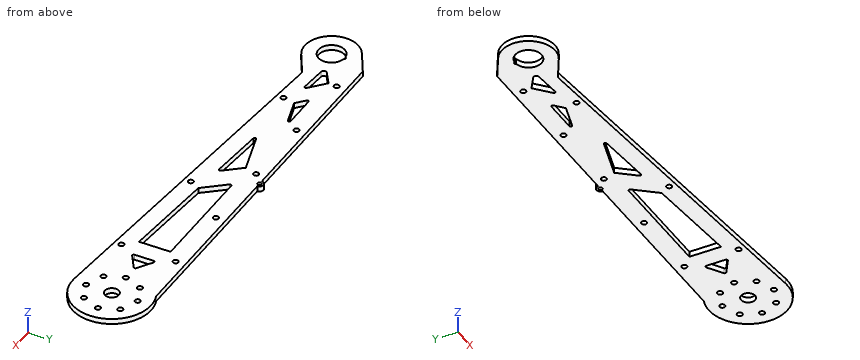
```python
from build123d import *

# Parameters (mm, degrees)
SKETCH_1_R          = 9.7
SKETCH_1_R_2        = 5.2
SKETCH_1_R_3        = 2
EXTRUDE_1_DEPTH     = 4
CUT_EXTRUDE_1_DEPTH = 10
SKETCH_3_R          = 3
EXTRUDE_2_DEPTH     = 4
SKETCH_4_R          = 1.5
CUT_EXTRUDE_2_DEPTH = 4
SKETCH_5_R          = 1
CUT_EXTRUDE_3_DEPTH = 10


with BuildPart() as part:
    # 草图1 → 凸台-拉伸1 (new body)
    with BuildSketch(Plane.XY):
        with BuildLine():
            Line((-9.85, 17.060700455), (7.470508076, 27.060700455))
            Line((7.470508076, 27.060700455), (289.624667154, 27.060700455))
            ThreePointArc((289.624667154, 27.060700455), (328.694852344, 4.11311011), (297.66555963, -28.905888469))
            Line((297.66555963, -28.905888469), (27.170508076, -7.060700455))
            Line((27.170508076, -7.060700455), (9.85, -17.060700455))
            ThreePointArc((9.85, -17.060700455), (-17.060700455, -9.85), (-9.85, 17.060700455))
        make_face()
        Circle(SKETCH_1_R, mode=Mode.SUBTRACT)
        with Locations((300, 0)):
            Circle(SKETCH_1_R_2, mode=Mode.SUBTRACT)
        with Locations((319, 0)):
            Circle(SKETCH_1_R_3, mode=Mode.SUBTRACT)
        with Locations((313.435028843, -13.435028843)):
            Circle(SKETCH_1_R_3, mode=Mode.SUBTRACT)
        with Locations((300, -19)):
            Circle(SKETCH_1_R_3, mode=Mode.SUBTRACT)
        with Locations((286.564971157, -13.435028843)):
            Circle(SKETCH_1_R_3, mode=Mode.SUBTRACT)
        with Locations((281, 0)):
            Circle(SKETCH_1_R_3, mode=Mode.SUBTRACT)
        with Locations((286.564971157, 13.435028843)):
            Circle(SKETCH_1_R_3, mode=Mode.SUBTRACT)
        with Locations((300, 19)):
            Circle(SKETCH_1_R_3, mode=Mode.SUBTRACT)
        with Locations((313.435028843, 13.435028843)):
            Circle(SKETCH_1_R_3, mode=Mode.SUBTRACT)
        with Locations((250, 20)):
            Circle(SKETCH_1_R_3, mode=Mode.SUBTRACT)
        with Locations((195, 20)):
            Circle(SKETCH_1_R_3, mode=Mode.SUBTRACT)
        with Locations((140, 20)):
            Circle(SKETCH_1_R_3, mode=Mode.SUBTRACT)
        with Locations((85, 20)):
            Circle(SKETCH_1_R_3, mode=Mode.SUBTRACT)
        with Locations((30, 20)):
            Circle(SKETCH_1_R_3, mode=Mode.SUBTRACT)
        with Locations(Location((250, -20, 0), (0, 0, 180))):
            Circle(SKETCH_1_R_3, mode=Mode.SUBTRACT)
        with Locations((167.5, -13.337297667)):
            Circle(SKETCH_1_R_3, mode=Mode.SUBTRACT)
        with Locations((57.5, -4.453694555)):
            Circle(SKETCH_1_R_3, mode=Mode.SUBTRACT)
    extrude(amount=EXTRUDE_1_DEPTH)

    # 草图2 → 切除-拉伸1 (cut)
    with BuildSketch(Plane(origin=(0, 0, 0), x_dir=(-1, 0, 0), z_dir=(0, 0, -1))):
        with BuildLine():
            Line((-137.197603441, 10.82531174), (-106.043706264, 1.591034337))
            ThreePointArc((-106.043706264, 1.591034337), (-105.333274422, 0.528665045), (-106.247395472, -0.364489265))
            Line((-106.247395472, -0.364489265), (-146.939942745, -3.650820533))
            ThreePointArc((-146.939942745, -3.650820533), (-147.907056702, -3.116572023), (-147.791851116, -2.017727835))
            Line((-147.791851116, -2.017727835), (-137.197603441, 10.82531174))
        make_face()
        with BuildLine():
            Line((-242, 12), (-159.091058121, 12))
            ThreePointArc((-159.091058121, 12), (-158.186531194, 11.426416508), (-158.319647694, 10.363662077))
            Line((-158.319647694, 10.363662077), (-171.517559676, -5.635709572))
            Line((-171.517559676, -5.635709572), (-242, -11.327873446))
            Line((-242, -11.327873446), (-242, 12))
        make_face()
        with BuildLine():
            Line((-77.967218715, 12), (-53.665101582, 12))
            ThreePointArc((-53.665101582, 12), (-52.730413268, 11.355468359), (-53.000597339, 10.252715509))
            Line((-53.000597339, 10.252715509), (-59.49167188, 4.480688084))
            Line((-59.49167188, 4.480688084), (-78.251405867, 10.041231173))
            ThreePointArc((-78.251405867, 10.041231173), (-78.956857242, 11.14358129), (-77.967218715, 12))
        make_face()
        with BuildLine():
            Line((-268.630020148, 0.840296648), (-257.54212687, 7.993776182))
            ThreePointArc((-257.54212687, 7.993776182), (-256.52152684, 8.031581712), (-256, 7.153479534))
            Line((-256, 7.153479534), (-256, -7.153479534))
            ThreePointArc((-256, -7.153479534), (-256.52152684, -8.031581712), (-257.54212687, -7.993776182))
            Line((-257.54212687, -7.993776182), (-268.630020148, -0.840296648))
            ThreePointArc((-268.630020148, -0.840296648), (-269.087893278, 0), (-268.630020148, 0.840296648))
        make_face()
        with BuildLine():
            Line((-19.631707517, 7.078552885), (-29.56189752, 13.698679554))
            Line((-29.56189752, 13.698679554), (-40.860283753, 3.651869157))
            ThreePointArc((-40.860283753, 3.651869157), (-41.116034111, 2.513264507), (-40.118555254, 1.907570918))
            Line((-40.118555254, 1.907570918), (-20.586659398, 3.4204248))
            ThreePointArc((-20.586659398, 3.4204248), (-18.805958358, 4.909282805), (-19.631707517, 7.078552885))
        make_face()
    extrude(amount=-CUT_EXTRUDE_1_DEPTH, mode=Mode.SUBTRACT)

    # 草图3 → 凸台-拉伸2 (add)
    with BuildSketch(Plane(origin=(0, 0, 0), x_dir=(-1, 0, 0), z_dir=(0, 0, -1))):
        with Locations((-148.547587615, 27.060700455)):
            Circle(SKETCH_3_R)
    extrude(amount=-EXTRUDE_2_DEPTH)

    # 草图4 → 切除-拉伸2 (cut)
    with BuildSketch(Plane(origin=(0, 0, 0), x_dir=(-1, 0, 0), z_dir=(0, 0, -1))):
        with Locations((-148.547587615, 27.060700455)):
            Circle(SKETCH_4_R)
    extrude(amount=-CUT_EXTRUDE_2_DEPTH, mode=Mode.SUBTRACT)

    # 草图5 → 切除-拉伸3 (cut)
    with BuildSketch(Plane(origin=(0, 0, 0), x_dir=(-1, 0, 0), z_dir=(0, 0, -1))):
        with Locations((0, 9.7)):
            Circle(SKETCH_5_R)
    extrude(amount=-CUT_EXTRUDE_3_DEPTH, mode=Mode.SUBTRACT)


solid = part.part
```
The listing builds one solid part. Answer for the finished solid, in the listing's coordinates (mm). Coordinates: 2 decimals unless noted, no trailing zeros. Loops run counter-clockwise (first coordinate to the right, second up) from the corner with the lowest first, then second, coordinate; pieces in that order, holes last. Notation, with made-up numbers: M -15.5,11 L -8.5,11 A28 ccw -8.5,35 Z; hole C 64,77 d4. An arc over 180 degrees is marked long. Answer as CSV lines item,"result". Start each with the question number.
(1) Find the intervals of material crossed by L1, parallel to Y at x = 57.5, z = 2.1; L2, parallel to Y at x = 30, z = 1.2; L3, parallel to Y at x = 163.5, z = 3.15, in increasing order. Write a range as [from, to].
(2) Given pin 1 (3 mm diameter, centred on x = 286.56, y = 13.44, fed in from +Z); pin 2 (1.5 mm diameter, centred on x = 79, z = 0.5, fed in from +Y), each flat-ended and moving along its own axis, determine where each tip first touches the part or whether it passes through.
(3) The part is cut by section D-D (x = 15). Give the vertices of the cut face in (y, z).
(4) The part is cut by section C-C (z = 0.75). State how many separate pieces and enclosed holes the cut face has, and give its area (3 significant figures).
(5) The part is cut by section B-B (x = 66). Give the vertices of the cut face in (y, z).
(6) The part is cut by section A-A (x = 177). Give the vertices of the cut face in (y, z).
Determined:
1,L1,"[-9.51, -6.45], [-2.45, 6.25], [12, 27.06]"
1,L2,"[-7.29, 2.69], [13.31, 18], [22, 27.06]"
1,L3,"[-18.07, 4.08], [12, 27.06]"
2,pin 1,"through"
2,pin 2,"y = 27.06"
3,outline,"M -14.09,0 L 27.06,0 L 27.06,4 L -14.09,4 Z"
4,separate pieces,"1"
4,enclosed holes,"24"
4,area,"12,500 mm2"
5,outline,"M -10.2,0 L 6.41,0 L 6.41,4 L -10.2,4 Z; M 12,0 L 27.06,0 L 27.06,4 L 12,4 Z"
6,outline,"M -19.16,0 L -6.08,0 L -6.08,4 L -19.16,4 Z; M 12,0 L 27.06,0 L 27.06,4 L 12,4 Z"
